Verification items for the finished model (mm, model axes). Face numbers are marked on the shaded views. Coordinates: 2 decimals unless noted, no trailing zeros. One line per question, with ' | ' between items. Start each with the question number.
from build123d import *

# Parameters (mm, degrees)
F0_R     = 114.3
F0_R_2   = 77.7875
F1_DEPTH = 6.35
F2_DEPTH = 203.2
F3_DEPTH = 101.6
F4_R     = 6.35
F5_DEPTH = 101.601
F6_T     = -2.54
F7_DEPTH = 9.525
F8_DEPTH = 25.4


# Not quite as in the source:
# - a shell that OpenCascade refuses in one call is made with other operations: the cavity is built on its own and cut out


with BuildPart() as f1:
    # F0 (on Front) → F1 (new body)
    with BuildSketch(Plane.XZ):
        Circle(F0_R)
        Circle(F0_R_2, mode=Mode.SUBTRACT)
    extrude(amount=F1_DEPTH)

    # F0 (on Front) → F2 (join)
    with BuildSketch(Plane.XZ):
        Circle(F0_R_2)
    extrude(amount=F2_DEPTH)

    # F3 (cut): a face of the model
    f3_faces = [f1.faces().sort_by_distance(p)[0] for p in [
        (0, -203.2, 0),
    ]]
    extrude(f3_faces, amount=-F3_DEPTH, mode=Mode.SUBTRACT)

    # F4 (on face) → F5 (cut, through all)
    with BuildSketch(Plane.XZ.offset(101.6)):
        Circle(F4_R)
    extrude(amount=-F5_DEPTH, mode=Mode.SUBTRACT)

    # F6: a shell. OpenCascade refuses it in one call, so the cavity is built on its own and cut out:
    # the body offset inwards by the wall thickness, plus a prism from it out through each open face.
    f6_core = offset(f1.part, amount=F6_T, kind=Kind.INTERSECTION, mode=Mode.PRIVATE)
    f6_exits = [f6_core.faces().sort_by_distance(p)[0] for p in [
        (-78.40855, -3.81, 0),
    ]]
    add(f6_core, mode=Mode.SUBTRACT)
    extrude(f6_exits, amount=-F6_T, mode=Mode.SUBTRACT)

    # F7 (add): a face of the model
    f7_faces = [f1.faces().sort_by_distance(p)[0] for p in [
        (-75.5873372503, -101.6, 0),
    ]]
    extrude(f7_faces, amount=F7_DEPTH)

    # F8 (add): a face of the model
    f8_faces = [f1.faces().sort_by_distance(p)[0] for p in [
        (-75.5873372503, -111.125, 0),
    ]]
    extrude(f8_faces, amount=F8_DEPTH)


solid = f1.part
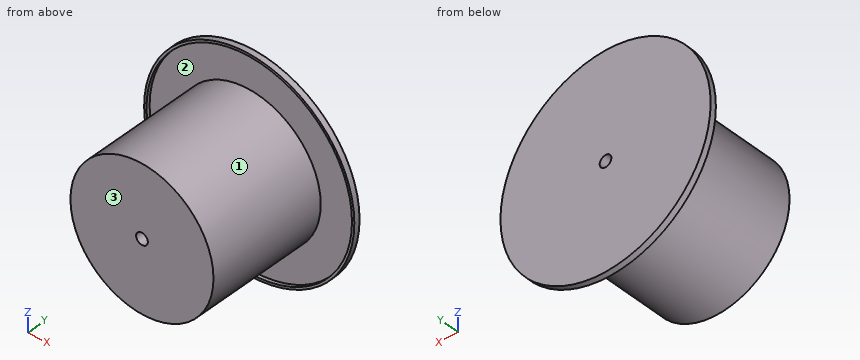
Item 1: Section check A-A (y = -35). Give the number of separate pieces and of enclosed holes in the cut face, then the cut area to 3 significant figures.
Item 2: Mould release check, pull along Z, two halves, no side actions. Record for the marked faces 1, 2 and 3: +Z half, -Z half, draft (parallel to the pull), parting line (faces both ways), or undercut.
Item 3: Gauge pin test, flat ends, axial feed: pin 1 (5 mm diameter, centred on x = 45, y = -66.5, fed in from +Z); pin 2 (1 mm diameter, centred on x = 10.5, y = -95, fed in from +Z); pin 3 (2 mm diameter, centred on x = -66, y = -85, fed in from -Z); pin 4 (11.5 mm diameter, centred on x = 0, z = 0, fed in from -Y). Record the tip position at first contact, or that the pin passes through.
Item 4: Thickness scan on probe 1 along Z at (x, y) = (0, -3.45); probe 2 along Z at (x, y) = (0, -108); probe 3 along Z at (x, y) = (0, -23). Record the ranges inside material, lowest first. Write a range as from..to.
Completed:
1) separate pieces: 2 | enclosed holes: 2 | area: 1,340 mm^2
2) face 1: parting line | face 2: undercut | face 3: draft
3) pin 1: stops at z = 65.15 | pin 2: stops at z = 77.14 | pin 3: stops at z = -42.73 | pin 4: passes through
4) probe 1: z = -114.3..-111.76, -8.89..-6.35, 6.35..8.89, 111.76..114.3 | probe 2: z = -77.79..-6.35, 6.35..77.79 | probe 3: z = -77.79..-75.25, -8.89..-6.35, 6.35..8.89, 75.25..77.79
